from build123d import *

# Parameters (mm, degrees)
SKETCH1_R           = 1.25
SKETCH1_R_2         = 4.85
SKETCH1_R_3         = 0.325511789
BOSS_EXTRUDE1_DEPTH = 1.6
BOSS_EXTRUDE2_START = 1.6
SKETCH1_3_R         = 4.85
BOSS_EXTRUDE2_DEPTH = 7.3
FILLET1_R           = 0.5
SKETCH2_R           = 4.35
BOSS_EXTRUDE3_DEPTH = 0.1


with BuildPart() as part:
    # Sketch1 → Boss-Extrude1 (new body)
    # profile 1 of 2: a face of its own
    with BuildSketch(Plane.XY):
        Polygon((0, 20.3), (1.4, 21.7), (12.6, 21.7), (14, 20.3), (14, 1.4), (12.6, 0), (1.4, 0), (0, 1.4), align=None)
        with Locations((2.05, 19.35)):
            Circle(SKETCH1_R, mode=Mode.SUBTRACT)
        with Locations((11.84, 19.35)):
            Circle(SKETCH1_R, mode=Mode.SUBTRACT)
        with Locations((7.55, 14.15)):
            Circle(SKETCH1_R_2, mode=Mode.SUBTRACT)
        with Locations((9.38, 1.5)):
            Circle(SKETCH1_R_3, mode=Mode.SUBTRACT)
        with Locations((6.84, 1.5)):
            Circle(SKETCH1_R_3, mode=Mode.SUBTRACT)
        with Locations((4.3, 1.5)):
            Circle(SKETCH1_R_3, mode=Mode.SUBTRACT)
    # profile 2 of 2: a face of its own
    with BuildSketch(Plane.XY):
        with Locations((7.55, 14.15)):
            Circle(SKETCH1_R_2)
    extrude(amount=BOSS_EXTRUDE1_DEPTH)

    # Sketch1<3> → Boss-Extrude2 (add)
    with BuildSketch(Plane.XY.offset(BOSS_EXTRUDE2_START)):
        with Locations((7.55, 14.15)):
            Circle(SKETCH1_3_R)
    extrude(amount=BOSS_EXTRUDE2_DEPTH)

    # Fillet1
    fillet1_edges = [part.edges().sort_by_distance(p)[0] for p in [
        (2.7, 14.15, 8.9),
    ]]
    fillet(fillet1_edges, radius=FILLET1_R)

    # Sketch2 → Boss-Extrude3 (add)
    with BuildSketch(Plane.XY.offset(8.9)):
        with Locations((7.55, 14.15)):
            Circle(SKETCH2_R)
    extrude(amount=BOSS_EXTRUDE3_DEPTH)


solid = part.part
Check sheet for the modelled part. Datum: model origin and axes. Units: mm. A direction names the side the tool comes from. Give positions to 0.01 mm unless a question says otherwise; leave off trailing zeros. Write each loop counter-clockwise with the first axis right and the second up, starting at its lowest first coordinate (ties: lowest second). Pieces come first, ordered by that corner, then holes. Notation, with made-up numbers: (42.25, 30) -> (61.25, 30) arc R5 cw to (61.25, 38) -> close; hole circle Ø7 at (89, -1). An arc over 180 degrees is marked (long way). Use one line per item in the form item = value. Start each with the question number.
1. Go/stop test with flat-tipped pins: P1, Ø1, axis at x = 12.5, z = 7, coming from the +Y side; P2, Ø5, axis at y = 11.5, z = 5, coming from the +X side; P3, Ø3, axis at x = 3, z = 8, coming from the +Y side. Record where each tip stops, or that it passes through.
2. Section check C-C (z = 1). Record the cut outline in (x, y), and give its area (3 significant figures).
3. Section check D-D (y = 14.15). Record the cut outline in (x, z).
4. Thickness scan on line 1 along Y through (x, z) = (11.84, 0.65); line 2 along Z through (x, y) = (0.5, 4); line 3 along Y through (x, z) = (7.5, 3). Record the ranges inside material, lowest first. Write a range as from..to.
5. Section check A-A (y = 19.35). Record the cut outline in (x, z).
6. Section check B-B (x = 7.55). Record the cut outline in (y, z).
7. Access from +Z, -Z, +X, -X, +Y, -Y to the whole of each face (thin tool, end or side, straight path). Record for faces 1 (the flat face through (7, 14, 9)), 2 (the cylindrical face through (10.16, 18.24, 4.95)).
Conclusion:
q1.P1 = 16.08
q1.P2 = 12.4
q1.P3 = 17.92
q2.outline = (0, 1.4) -> (1.4, 0) -> (12.6, 0) -> (14, 1.4) -> (14, 20.3) -> (12.6, 21.7) -> (1.4, 21.7) -> (0, 20.3) -> close; hole circle Ø2.5 at (2.05, 19.35); hole circle Ø0.65 at (4.3, 1.5); hole circle Ø0.65 at (6.84, 1.5); hole circle Ø0.65 at (9.38, 1.5); hole circle Ø2.5 at (11.84, 19.35)
q2.area = 289 mm²
q3.outline = (0, 0) -> (14, 0) -> (14, 1.6) -> (12.4, 1.6) -> (12.4, 8.4) arc R0.5 ccw to (11.9, 8.9) -> (11.9, 9) -> (3.2, 9) -> (3.2, 8.9) arc R0.5 ccw to (2.7, 8.4) -> (2.7, 1.6) -> (0, 1.6) -> close
q4.line_1 = 0..18.1, 20.6..21.7
q4.line_2 = 0..1.6
q4.line_3 = 9.3..19
q5.outline = (0, 0) -> (0.8, 0) -> (0.8, 1.6) -> (0, 1.6) -> close; (3.3, 0) -> (10.59, 0) -> (10.59, 1.6) -> (3.3, 1.6) -> close; (13.09, 0) -> (14, 0) -> (14, 1.6) -> (13.09, 1.6) -> close
q6.outline = (0, 0) -> (21.7, 0) -> (21.7, 1.6) -> (19, 1.6) -> (19, 8.4) arc R0.5 ccw to (18.5, 8.9) -> (18.5, 9) -> (9.8, 9) -> (9.8, 8.9) arc R0.5 ccw to (9.3, 8.4) -> (9.3, 1.6) -> (0, 1.6) -> close
q7.face_1 = +Z, +X, -X, +Y, -Y
q7.face_2 = +Z
